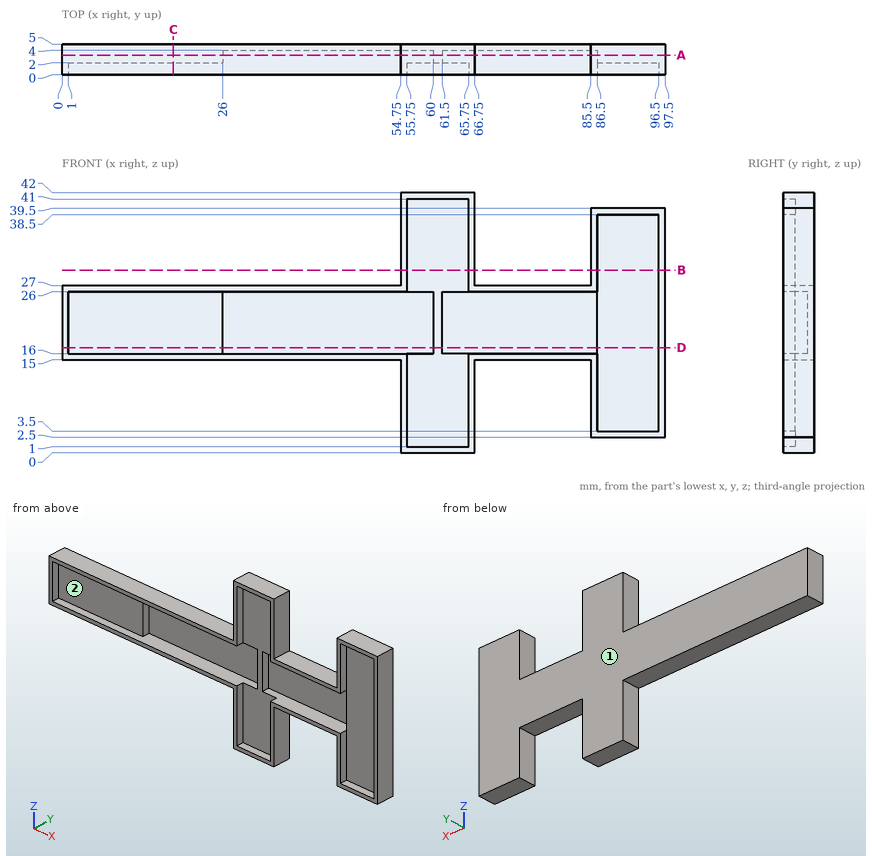
Verification items for this drawing (mm, ordinates from the low corner). Coordinates: 2 decimals unless noted, no trailing zeros. Write each loop counter-clockwise with the first axis right and the second up, starting at its lowest first coordinate (ties: lowest second). Pieces come first, ordered by that corner, then holes. Notation, with made-up numbers: (68, 77) -> (93, 77) arc R19 cw to (93, 82) -> close; hole circle Ø10 at (42, 34). An arc over 180 degrees is marked (long way). One line per item, written item: value. Start each with the question number.
Q1. Cross-section at C-C on x = 18. Enter the section's corners in (y, z).
Q2. Cross-section at A-A on y = 3.2. Enter the section's corners in (x, z).
Q3. Cross-section at B-B on z = 29.5. Enter the section's corners in (x, y), and give its area (3 significant figures).
Q4. Thickness scan on L1, parallel to X at y = 3.9, z = 20.5; L2, parallel to X at y = 4.3, z = 11; L3, parallel to Z at x = 77.5, y = 1.35. Record the ranges inside material, lowest first. Write a range as from..to.
Q5. Cross-section at D-D on z = 17. Enter the section's corners in (x, y), and give its area (4 significant figures).
Q6. Mould release check, pull along Z, two halves, no side actions. Record for the marked faces 1 and 2: pulls with the +Z half, pulls with the -Z half, needs draft (parallel to the pull), parting line crosses it, or undercut.
Q7. Go/stop test with flat-tipped pins: P1, Ø1, axis at x = 31.5, y = 2.5, coming from the -Z side; P2, Ø2.5, axis at y = 3, z = 30, coming from the -X side; P3, Ø2, axis at x = 89, y = 1, coming from the -Z side. Record where each tip stops, or that it passes through.
Checked values:
1. outline: (0, 15) -> (5, 15) -> (5, 27) -> (0, 27) -> (0, 26) -> (2, 26) -> (2, 16) -> (0, 16) -> close
2. outline: (0, 15) -> (54.75, 15) -> (54.75, 0) -> (66.75, 0) -> (66.75, 15) -> (85.5, 15) -> (85.5, 2.5) -> (97.5, 2.5) -> (97.5, 39.5) -> (85.5, 39.5) -> (85.5, 27) -> (66.75, 27) -> (66.75, 42) -> (54.75, 42) -> (54.75, 27) -> (0, 27) -> close; hole (26, 16) -> (60, 16) -> (60, 26) -> (26, 26) -> close; hole (61.5, 16) -> (86.5, 16) -> (86.5, 26) -> (61.5, 26) -> close
3. outline: (54.75, 0) -> (55.75, 0) -> (55.75, 2) -> (65.75, 2) -> (65.75, 0) -> (66.75, 0) -> (66.75, 5) -> (54.75, 5) -> close; (85.5, 0) -> (86.5, 0) -> (86.5, 2) -> (96.5, 2) -> (96.5, 0) -> (97.5, 0) -> (97.5, 5) -> (85.5, 5) -> close
3. area: 80.0 mm²
4. L1: x = 0..26, 60..61.5, 86.5..97.5
4. L2: x = 54.75..66.75, 85.5..97.5
4. L3: z = 15..16, 26..27
5. outline: (0, 0) -> (1, 0) -> (1, 2) -> (26, 2) -> (26, 4) -> (60, 4) -> (60, 2) -> (61.5, 2) -> (61.5, 4) -> (86.5, 4) -> (86.5, 2) -> (96.5, 2) -> (96.5, 0) -> (97.5, 0) -> (97.5, 5) -> (0, 5) -> close
5. area: 178.5 mm²
6. face 1: needs draft
6. face 2: undercut
7. P1: stops at z = 15
7. P2: stops at x = 54.75
7. P3: stops at z = 2.5
